from build123d import *

# Parameters (mm, degrees)
BOSS_EXTRUDE2_DEPTH      = 50
BOSS_EXTRUDE2_DEPTH_BACK = 50
CUT_EXTRUDE2_DEPTH       = 209.62646045
BOSS_EXTRUDE3_DEPTH      = 35
BOSS_EXTRUDE3_DEPTH_BACK = 35
SKETCH10_W               = 99.044902454
SKETCH10_H               = 40
CUT_EXTRUDE3_DEPTH       = 179.937459443


with BuildPart() as part:
    # Sketch1 → Boss-Extrude2 (new, two sides: drawn at the far end of the back side and taken through both)
    with BuildSketch(Plane.XY.offset(-BOSS_EXTRUDE2_DEPTH_BACK)):
        with BuildLine():
            Line((0, 0), (150, 0))
            Line((150, 0), (150, 21.222828934))
            Line((150, 21.222828934), (50, 21.222828934))
            Line((50, 21.222828934), (50, 80))
            ThreePointArc((50, 80), (25, 105), (0, 80))
            Line((0, 80), (0, 0))
        make_face()
    extrude(amount=BOSS_EXTRUDE2_DEPTH + BOSS_EXTRUDE2_DEPTH_BACK)

    # Sketch7 → Cut-Extrude2 (cut, through all)
    with BuildSketch(Plane.XY.offset(50)):
        with BuildLine():
            Line((35, 80), (35, 25))
            ThreePointArc((35, 25), (25, 15), (15, 25))
            Line((15, 25), (15, 80))
            ThreePointArc((15, 80), (25, 90), (35, 80))
        make_face()
    extrude(amount=-CUT_EXTRUDE2_DEPTH, mode=Mode.SUBTRACT)

    # Sketch9 → Boss-Extrude3 (add, two sides: drawn at the far end of the back side and taken through both)
    with BuildSketch(Plane.XY.offset(-BOSS_EXTRUDE3_DEPTH_BACK)):
        Polygon((50, 66.222828934), (50, 21.222828934), (140, 21.222828934), align=None)
    extrude(amount=BOSS_EXTRUDE3_DEPTH + BOSS_EXTRUDE3_DEPTH_BACK)

    # Sketch10 → Cut-Extrude3 (cut, through all)
    with BuildSketch(Plane(origin=(0, 21.222828934, 0), x_dir=(1, 0, 0), z_dir=(0, 1, 0))):
        with Locations((99.522451227, 0)):
            Rectangle(SKETCH10_W, SKETCH10_H)
    extrude(amount=CUT_EXTRUDE3_DEPTH, mode=Mode.SUBTRACT)


solid = part.part
Design review of the part built by this model. Coordinates are the model's own, in mm. A direction names the side the tool comes from. Coordinates: 2 decimals unless noted, no trailing zeros. Order: outer loops, then holes, each group sorted by start corner. A loop starts at its lowest first (then second) coordinate and runs counter-clockwise, first axis right, second up. Notation, with made-up numbers: (-24, 22.5) - (26, 22.5) arc R16 cw to (26, 44.5) - close; hole circle Ø5 at (40, 81.5). An arc over 180 degrees is marked (long way). Put each result on its own line as item: value.
1) Tool access review of faces 4 (the face through (101, 21.223, -1)), 5 (the face through (25, 90, 1)), 6 (the face through (0, 41, -1)): name each direction out of +Z, -Z, +X, -X, +Y, -Y from which nothing blocks a thin tool from reaching the whole face with its end or side.
Response values:
face 4: +X, +Y
face 5: +Z, -Z
face 6: +Z, -Z, -X, +Y, -Y
2) The part is to be moulded in two halves that separate along Z. For faces 1 (the face through (74, 34, 35)), 2 (the face through (74, 34, -35)), 3 (the face through (84, 38, -20)), say which applies: released by +Z, released by -Z, zero draft, split by the parting line, or undercut.
Response values:
face 1: released by +Z
face 2: released by -Z
face 3: undercut
3) Take a section at A-A, the plane x = 25. Give the boundary of the cut face in (y, z), and give its area (3 significant figures).
Response values:
outline: (0, -50) - (15, -50) - (15, 50) - (0, 50) - close; (90, -50) - (105, -50) - (105, 50) - (90, 50) - close
area: 3,000 mm²
4) Wall thickness on L1, parallel to X at y = 64.5, z = 38; L2, parallel to Y at x = 53, z = 8.5; L3, parallel to Z at x = 71, y = 23: over which ranges is each line inside the solid? List them lowest first. Write a range as from..to.
Response values:
L1: x = 0..15, 35..50
L2: y = 0..21.22
L3: z = -35..-20, 20..35
5) Insertion check: P1, Ø17.5, axis at y = 54, z = -23, coming from the +X side; P2, Ø6, axis at x = 111, z = 6.5, coming from the +Y side; P3, Ø12, axis at y = 86, z = 3.5, coming from the +X side. Each pin has a flat end and moves straight along its axis. Give the tip position at first contact, or say it passes through.
Response values:
P1: stops at x = 91.95
P2: stops at y = 21.22
P3: stops at x = 50
6) Take a section at B-B, the plane z = 38. Give the boundary of the cut face in (x, y).
Response values:
outline: (0, 0) - (150, 0) - (150, 21.22) - (50, 21.22) - (50, 80) arc R25 ccw to (0, 80) - close; hole (15, 25) arc R10 ccw to (35, 25) - (35, 80) arc R10 ccw to (15, 80) - close
7) Take a section at D-D, the plane x = 118. Give the boundary of the cut face in (y, z).
Response values:
outline: (0, -50) - (21.22, -50) - (21.22, -35) - (32.22, -35) - (32.22, -20) - (21.22, -20) - (21.22, 20) - (32.22, 20) - (32.22, 35) - (21.22, 35) - (21.22, 50) - (0, 50) - close
8) Take a section at C-C, the plane y = 68. Give the boundary of the cut face in (x, z).
Response values:
outline: (0, -50) - (15, -50) - (15, 50) - (0, 50) - close; (35, -50) - (50, -50) - (50, 50) - (35, 50) - close
